```python
from build123d import *

# Parameters (mm, degrees)
BOSS_EXTRUDE1_DEPTH                              = 40
CHAMFER1_SIZE                                    = 7
FILLET1_R                                        = 3
CBORE_FOR_M4_PAN_HEAD_MACHINE_SCREW1_D           = 4.3
CBORE_FOR_M4_PAN_HEAD_MACHINE_SCREW1_DEPTH       = 5.5
CBORE_FOR_M4_PAN_HEAD_MACHINE_SCREW1_CBORE_D     = 9
CBORE_FOR_M4_PAN_HEAD_MACHINE_SCREW1_CBORE_DEPTH = 3.1


with BuildPart() as part:
    # Sketch1 → Boss-Extrude1 (new body)
    with BuildSketch(Plane.XY):
        Polygon((0, 32), (0, -32), (-40, -32), (-40, -28), (-4.5, -28), (-4.5, 26.5), (-60, 26.5), (-60, 32), align=None)
    extrude(amount=BOSS_EXTRUDE1_DEPTH)

    # Chamfer1
    chamfer1_edges = [part.edges().sort_by_distance(p)[0] for p in [
        (-4.5, -28, 20),
        (-4.5, 26.5, 20),
    ]]
    chamfer(chamfer1_edges, length=CHAMFER1_SIZE)

    # Fillet1
    fillet1_edges = [part.edges().sort_by_distance(p)[0] for p in [
        (-60, 32, 20),
        (0, 32, 20),
        (0, -32, 20),
        (-11.5, -28, 20),
        (-4.5, 19.5, 20),
        (-4.5, -21, 20),
        (-11.5, 26.5, 20),
    ]]
    fillet(fillet1_edges, radius=FILLET1_R)

    # CBORE for M4 Pan Head Machine Screw1
    with Locations(Plane(origin=(0, 32, 0), x_dir=(1, 0, 0), z_dir=(0, 1, 0))):
        with Locations((-53, -11), (-53, -29), (-29, -29), (-29, -11)):
            CounterBoreHole(CBORE_FOR_M4_PAN_HEAD_MACHINE_SCREW1_D / 2, CBORE_FOR_M4_PAN_HEAD_MACHINE_SCREW1_CBORE_D / 2, CBORE_FOR_M4_PAN_HEAD_MACHINE_SCREW1_CBORE_DEPTH, depth=CBORE_FOR_M4_PAN_HEAD_MACHINE_SCREW1_DEPTH)


solid = part.part
```
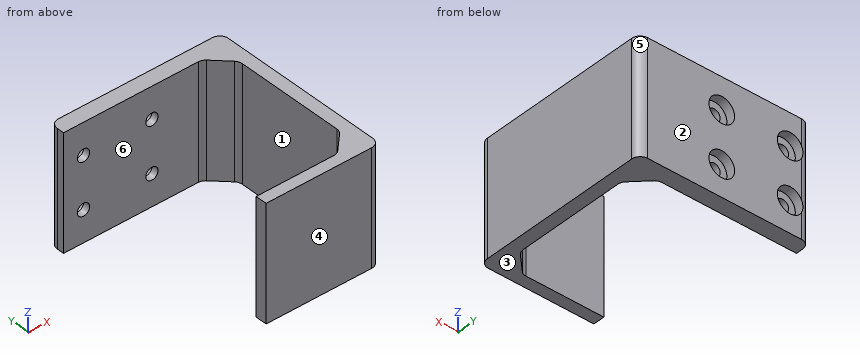
For this review, take the finished solid that the model builds, in its own axes (mm). Face numbers are marked on the shaded views. A direction names the side the tool comes from. Coordinates: 2 decimals unless noted, no trailing zeros. Write each loop counter-clockwise with the first axis right and the second up, starting at its lowest first coordinate (ties: lowest second). Pieces come first, ordered by that corner, then holes. Notation, with made-up numbers: (72.5, 22.5) -> (107.5, 22.5) arc R27 ccw to (107.5, 45.5) -> close; hole circle Ø5 at (48, -22.75). An arc over 180 degrees is marked (long way). Put each result on its own line as item: value.
Q1. Take a section at A-A, the plane x = -36. State the section outline as (y, z) points.
From the geometry:
outline: (-32, 0) -> (-28, 0) -> (-28, 40) -> (-32, 40) -> close; (26.5, 0) -> (32, 0) -> (32, 40) -> (26.5, 40) -> close
Q2. Wall thickness on L1, parallel to Z at x = -53, y = 31; L2, parallel to X at y = 27.5, z = 11; L3, parallel to Z at x = -29, y = 28: over which ranges is each line inside the solid? List them lowest first.
From the geometry:
L1: z = 0 to 6.5, 15.5 to 24.5, 33.5 to 40
L2: x = -60 to -55.15, -50.85 to -31.15, -26.85 to 0
L3: z = 0 to 8.85, 13.15 to 26.85, 31.15 to 40
Q3. Take a section at B-B, the plane x = -53. State the section outline as (y, z) points, then the cut area to 3 significant figures.
From the geometry:
outline: (26.5, 0) -> (32, 0) -> (32, 6.5) -> (28.9, 6.5) -> (28.9, 8.85) -> (26.5, 8.85) -> close; (26.5, 13.15) -> (28.9, 13.15) -> (28.9, 15.5) -> (32, 15.5) -> (32, 24.5) -> (28.9, 24.5) -> (28.9, 26.85) -> (26.5, 26.85) -> close; (26.5, 31.15) -> (28.9, 31.15) -> (28.9, 33.5) -> (32, 33.5) -> (32, 40) -> (26.5, 40) -> close
area: 144 mm2
Q4. The part is to be moulded in two halves that separate along Y. For the marked faces 3, 4, 5 and 6, say which applies: +Y half, -Y half, draft (parallel to the pull), parting line (faces both ways), or undercut.
From the geometry:
face 3: draft
face 4: -Y half
face 5: +Y half
face 6: undercut
Q5. Take a section at C-C, the plane z = 29. Count the separate pieces of the cut face and the enclosed holes in it, then the cut area to 3 significant figures.
From the geometry:
separate pieces: 3
enclosed holes: 0
area: 703 mm2
Q6. Take a section at D-D, the plane x = -29. State the section outline as (y, z) points.
From the geometry:
outline: (-32, 0) -> (-28, 0) -> (-28, 40) -> (-32, 40) -> close; (26.5, 0) -> (32, 0) -> (32, 6.5) -> (28.9, 6.5) -> (28.9, 8.85) -> (26.5, 8.85) -> close; (26.5, 13.15) -> (28.9, 13.15) -> (28.9, 15.5) -> (32, 15.5) -> (32, 24.5) -> (28.9, 24.5) -> (28.9, 26.85) -> (26.5, 26.85) -> close; (26.5, 31.15) -> (28.9, 31.15) -> (28.9, 33.5) -> (32, 33.5) -> (32, 40) -> (26.5, 40) -> close
Q7. Tool access review of the marked faces 1 and 2: name each direction out of +Z, -Z, +X, -X, +Y, -Y from which nothing blocks a thin tool from reaching the whole face with its end or side.
From the geometry:
face 1: +Z, -Z, -X
face 2: +Z, -Z, +X, -X, +Y
Q8. Clearance check with flat-ended pins moving along their axes: pin 1 Ø5.5 at (x, z) = (-29, 29) entering from +Y; pin 2 Ø2.5 at (x, z) = (-53, 29) entering from -Y; pin 3 Ø3 at (y, z) = (-19, 22.5) entering from -X; pin 4 Ø1.2 at (y, z) = (-29, 10.5) entering from -X. State where each tip first meets the part, or that it passes through.
From the geometry:
pin 1: stops at y = 28.9
pin 2: passes through
pin 3: stops at x = -4.59
pin 4: stops at x = -40
